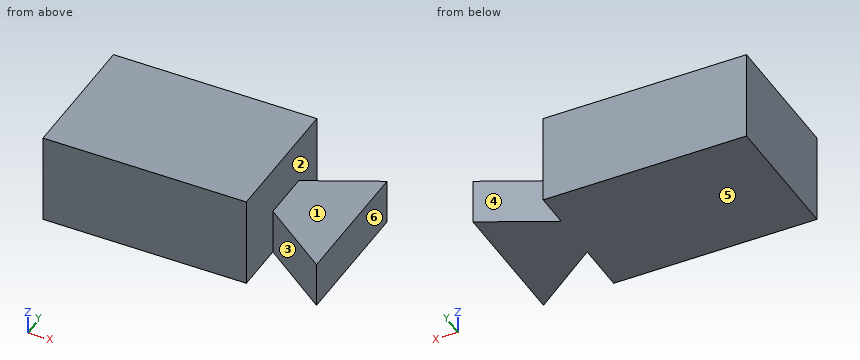
```python
from build123d import *

# Parameters (mm, degrees)
F0_W     = 152.4
F0_H     = 50.8
F1_DEPTH = 76.2
F3_DEPTH = 50.801
F4_W     = 48.462587264
F4_H     = 25.4
F5_DEPTH = 61.4661735057
F8_DEPTH = 25.4


with BuildPart() as f1:
    # F0 (on Front) → F1 (new body)
    with BuildSketch(Plane.XZ):
        with Locations((2.3709694028, -11.726943469)):
            Rectangle(F0_W, F0_H)
    extrude(amount=F1_DEPTH)

    # F2 (on face) → F3 (cut, through all)
    with BuildSketch(Plane.XY.offset(13.673056531)):
        Polygon((39.4796133041, -76.2), (78.5709694028, -76.2), (39.4796133041, -47.5558340549), align=None)
        Polygon((39.4796133041, 0), (39.4796133041, -19.5033811033), (78.5709694028, 0), align=None)
    extrude(amount=-F3_DEPTH, mode=Mode.SUBTRACT)

    # F4 (on face) → F5 (cut, through all)
    with BuildSketch(Plane(origin=(-8.8807709948, -12.1197936799, 0), x_dir=(0.8066295736, -0.5910572993, 0), z_dir=(-0.5910572993, -0.8066295736, 0))):
        with Locations((84.1849401183, 0.973056531)):
            Rectangle(F4_W, F4_H)
    extrude(amount=-F5_DEPTH, mode=Mode.SUBTRACT)

    # F7 (on face) → F8 (cut)
    with BuildSketch(Plane.XY.offset(13.673056531)):
        Polygon((39.4796133041, -19.5033811033), (39.4796133041, -47.5558340549), (71.8800364079, -3.338226891), align=None)
        Polygon((71.8800364079, -3.338226891), (39.4796133041, -47.5558340549), (60.0389204919, -83.1656008959), (93.497350812, -40.1085205376), align=None)
    extrude(amount=-F8_DEPTH, mode=Mode.SUBTRACT)


solid = f1.part
```
Check sheet for the modelled part. Datum: model origin and axes. Units: mm. Face numbers are marked on the shaded views. A direction names the side the tool comes from. Give positions to 0.01 mm unless a question says otherwise; leave off trailing zeros. Write each loop counter-clockwise with the first axis right and the second up, starting at its lowest first coordinate (ties: lowest second). Pieces come first, ordered by that corner, then holes. Notation, with made-up numbers: (63.5, 32.5) -> (120.5, 32.5) arc R17 cw to (120.5, 65.5) -> close; hole circle Ø4 at (6, -3.5). An arc over 180 degrees is marked (long way). Use CSV: the item, a comma, the result in double quotes. Start each with the question number.
Q1. Tool access check on the marked faces 1, 2 and 3. Record the directions out of +Z, -Z, +X, -X, +Y, -Y that give a thin tool (end or side, any length) a straight path to the whole face; none if there is none.
Q2. Release check for a two-part mould opening along X. For the marked faces 4, 5 and 6 record: +X half, -X half, draft (parallel to the pull), parting line (faces both ways), or undercut.
Q3. Cross-section at A-A on z = -25.5. Enter the section's corners in (x, y), and give its area (3 significant figures).
Q4. Depth check by flat-ended pin: P1, Ø3, axis at y = -64.5, z = 1, coming from the +X side; P2, Ø2, axis at x = 61, y = -62, coming from the +Z side; P3, Ø1, axis at x = 60.5, z = -15, coming from the +Y side. Enter the tip coordinate at first touch or a pass-through.
Q5. Cross-section at B-B on y = -70.5. Enter the section's corners in (x, z).
Q6. Cross-section at C-C on y = -21. Enter the section's corners in (x, z).
Q7. Scan lines: line 1 along X through (y, z) = (-4, 11); line 2 along Z through (x, y) = (50, -28.5); line 3 along X through (y, z) = (-8, -25). Record each from-to range of solid material in increasing order.
Q8. Cross-section at D-D on y = -60.5. Enter the section's corners in (x, z), and give its area (3 significant figures).
Working result:
1,face 1,"+Z, +X, +Y, -Y"
1,face 2,"+Z"
1,face 3,"+Z, -Z, -Y"
2,face 4,"undercut"
2,face 5,"draft"
2,face 6,"+X half"
3,outline,"(-73.83, -76.2) -> (39.48, -76.2) -> (39.48, -47.56) -> (78.57, -76.2) -> (78.57, 0) -> (39.48, -19.5) -> (39.48, 0) -> (-73.83, 0) -> close"
3,area,"10,700 mm^2"
4,P1,"stops at x = 39.48"
4,P2,"stops at z = -11.73"
4,P3,"stops at y = -8.77"
5,outline,"(-73.83, -37.13) -> (39.48, -37.13) -> (39.48, 13.67) -> (-73.83, 13.67) -> close; (70.79, -37.13) -> (78.57, -37.13) -> (78.57, -11.73) -> (70.79, -11.73) -> close"
6,outline,"(-73.83, -37.13) -> (78.57, -37.13) -> (78.57, -11.73) -> (39.48, -11.73) -> (39.48, 13.67) -> (-73.83, 13.67) -> close"
7,line 1,"x = -73.83 to 39.48"
7,line 2,"z = -37.13 to -11.73"
7,line 3,"x = -73.83 to 39.48, 62.54 to 78.57"
8,outline,"(-73.83, -37.13) -> (39.48, -37.13) -> (39.48, 13.67) -> (-73.83, 13.67) -> close; (57.14, -37.13) -> (78.57, -37.13) -> (78.57, -11.73) -> (57.14, -11.73) -> close"
8,area,"6,300 mm^2"
